The model under review builds one solid part; all positions refer to its coordinate system, in mm. Face numbers are marked on the shaded views. A direction names the side the tool comes from. Coordinates: 2 decimals unless noted, no trailing zeros. Write each loop counter-clockwise with the first axis right and the second up, starting at its lowest first coordinate (ties: lowest second). Pieces come first, ordered by that corner, then holes. Notation, with made-up numbers: (31.25, 59) - (45.25, 59) arc R23 cw to (45.25, 86) - close; hole circle Ø5 at (-27, 75). An arc over 180 degrees is marked (long way). Use one line per item in the form item = value. Start each with the question number.
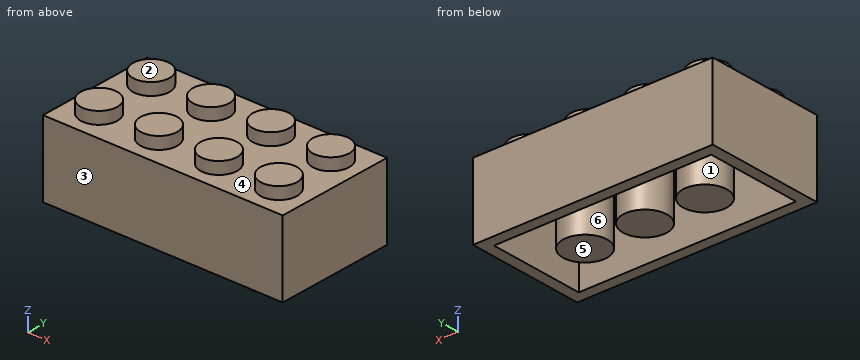
```python
from build123d import *

# Parameters (mm, degrees)
F0_W     = 32
F0_H     = 16
F1_DEPTH = 10
F2_T     = -1.5
F3_R     = 2.425
F4_DEPTH = 1.6
F5_R     = 2.925
F6_DEPTH = 10


with BuildPart() as f1:
    # F0 (on Top) → F1 (new body)
    with BuildSketch(Plane.XY):
        Rectangle(F0_W, F0_H)
    extrude(amount=F1_DEPTH)

    # F2
    f2_openings = [f1.faces().sort_by_distance(p)[0] for p in [
        (0, 0, 0),
    ]]
    offset(amount=F2_T, openings=f2_openings)

    # F3 (on face) → F4 (join)
    with BuildSketch(Plane.XY.offset(10)):
        with Locations((-12, -4)):
            Circle(F3_R)
        with Locations((-12, 4)):
            Circle(F3_R)
        with Locations((-4, -4)):
            Circle(F3_R)
        with Locations((-4, 4)):
            Circle(F3_R)
        with Locations((4, -4)):
            Circle(F3_R)
        with Locations((4, 4)):
            Circle(F3_R)
        with Locations((12, -4)):
            Circle(F3_R)
        with Locations((12, 4)):
            Circle(F3_R)
    extrude(amount=F4_DEPTH)

    # F5 (on face) → F6 (join)
    with BuildSketch(Plane.XY.offset(10)):
        with Locations((-8, 0)):
            Circle(F5_R)
        Circle(F5_R)
        with Locations((8, 0)):
            Circle(F5_R)
    extrude(amount=-F6_DEPTH)


solid = f1.part
```
1. Take a section at D-D (x = 0). State the section outline as (y, z) points (3 decimals), plus the area to 3 significant figures.
2. For P1, Ø1.5, axis at x = 1.5, y = -1, coming from the +Z side; P2, Ø1, axis at x = 8.5, y = 3.5, coming from the -Z side, all flat-tipped, find the tip position at first contact; note any pin that passes through.
3. For the marked faces 4, 5 and 6, list the 3-axis set-ups (+Z, -Z, +X, -X, +Y, -Y) from which the entire face can be reached by the end or side of a thin tool; tool diameter is ignored.
4. For L1, parallel to Y at x = -1, z = 4.75; L2, parallel to Y at x = 5, z = 7; L3, parallel to Y at x = -10.5, z = 5.25, list the stretches that pass through material, from the lowest coordinate up.
5. Take a section at C-C (x = 12). State the section outline as (y, z) points (3 decimals).
6. Take a section at B-B (y = 4). State the section outline as (x, z) points (3 decimals).
7. Take a section at A-A (z = 7.75). State the section outline as (x, y) points (3 decimals), plus the area to 3 significant figures.
8. The part is to be moulded in two halves that separate along Y. For the marked faces 1, 2 and 3, say which applies: released by +Y, released by -Y, zero draft, split by the parting line, or undercut.
Returned:
q1.outline = (-8, 0) - (-6.5, 0) - (-6.5, 8.5) - (-2.925, 8.5) - (-2.925, 0) - (2.925, 0) - (2.925, 8.5) - (6.5, 8.5) - (6.5, 0) - (8, 0) - (8, 10) - (-8, 10) - close
q1.area = 99.2 mm²
q2.P1 = 10
q2.P2 = 8.5
q3.face_4 = +Z
q3.face_5 = -Z, +X, -X, +Y, -Y
q3.face_6 = -Z
q4.L1 = -8 to -6.5, -2.75 to 2.75, 6.5 to 8
q4.L2 = -8 to -6.5, 6.5 to 8
q4.L3 = -8 to -6.5, -1.52 to 1.52, 6.5 to 8
q5.outline = (-8, 0) - (-6.5, 0) - (-6.5, 8.5) - (6.5, 8.5) - (6.5, 0) - (8, 0) - (8, 10) - (6.425, 10) - (6.425, 11.6) - (1.575, 11.6) - (1.575, 10) - (-1.575, 10) - (-1.575, 11.6) - (-6.425, 11.6) - (-6.425, 10) - (-8, 10) - close
q6.outline = (-16, 0) - (-14.5, 0) - (-14.5, 8.5) - (14.5, 8.5) - (14.5, 0) - (16, 0) - (16, 10) - (14.425, 10) - (14.425, 11.6) - (9.575, 11.6) - (9.575, 10) - (6.425, 10) - (6.425, 11.6) - (1.575, 11.6) - (1.575, 10) - (-1.575, 10) - (-1.575, 11.6) - (-6.425, 11.6) - (-6.425, 10) - (-9.575, 10) - (-9.575, 11.6) - (-14.425, 11.6) - (-14.425, 10) - (-16, 10) - close
q7.outline = (-16, -8) - (16, -8) - (16, 8) - (-16, 8) - close; circle Ø5.85 at (-8, 0); circle Ø5.85 at (0, 0); circle Ø5.85 at (8, 0); hole (-14.5, -6.5) - (14.5, -6.5) - (14.5, 6.5) - (-14.5, 6.5) - close
q7.area = 216 mm²
q8.face_1 = undercut
q8.face_2 = zero draft
q8.face_3 = released by -Y
